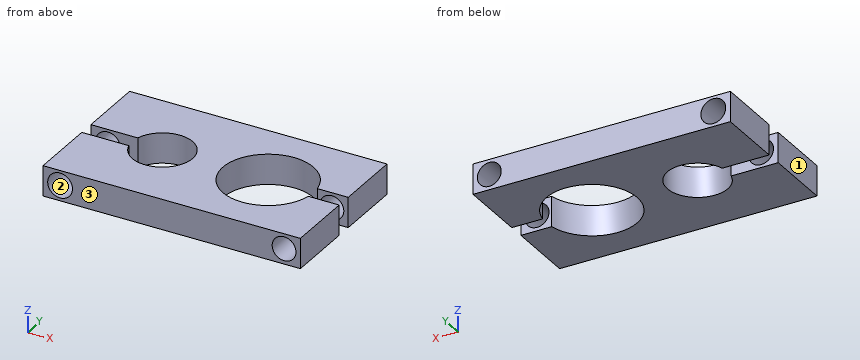
```python
from build123d import *

# Parameters (mm, degrees)
F1_DEPTH = 6.35
F2_R     = 2.607483
F2_R_2   = 2.505418
F3_DEPTH = 34.29


with BuildPart() as f1:
    # F0 (on Top) → F1 (new body)
    with BuildSketch(Plane.XY):
        with BuildLine():
            Line((27.051, 15.875), (-27.051, 15.875))
            Line((-27.051, 15.875), (-27.051, 1.651))
            Line((-27.051, 1.651), (-17.180615, 1.651))
            ThreePointArc((-17.180615, 1.651), (-4.699, 0), (-17.180615, -1.651))
            Line((-17.180615, -1.651), (-27.051, -1.651))
            Line((-27.051, -1.651), (-27.051, -15.875))
            Line((-27.051, -15.875), (27.051, -15.875))
            Line((27.051, -15.875), (27.051, -1.651))
            Line((27.051, -1.651), (20.556822, -1.651))
            ThreePointArc((20.556822, -1.651), (1.651, 0), (20.556822, 1.651))
            Line((20.556822, 1.651), (27.051, 1.651))
            Line((27.051, 1.651), (27.051, 15.875))
        make_face()
    extrude(amount=F1_DEPTH)

    # F2 (on face) → F3 (cut)
    with BuildSketch(Plane.XZ.offset(15.875)):
        with Locations((-23.459613, 3.213262)):
            Circle(F2_R)
        with Locations((23.626484, 3.213262)):
            Circle(F2_R_2)
    extrude(amount=-F3_DEPTH, mode=Mode.SUBTRACT)


solid = f1.part
```
Design review of the part built by this model. Coordinates are the model's own, in mm. Face numbers are marked on the shaded views. Coordinates: 2 decimals unless noted, no trailing zeros. Order: outer loops, then holes, each group sorted by start corner. A loop starts at its lowest first (then second) coordinate and runs counter-clockwise, first axis right, second up. Notation, with made-up numbers: (42, 56.25) -> (70, 56.25) arc R16 ccw to (70, 73.25) -> close; hole circle Ø6 at (44, 85.5). An arc over 180 degrees is marked (long way). One line per item, written item: value. Start each with the question number.
Q1. Take a section at A-A, the plane y = -9. State the section outline as (x, z) points, then the cut area to 3 significant figures.
Q2. Insertion check: pin 1 Ø3 at (x, y) = (-11, -4.5) entering from -Z. The pin has a flat end and moves straight along its axis. Give the tip position at first contact, or say it passes through.
Q3. Mouldability with a two-part tool opening along X and no side actions: class the marked faces 1, 2 and 3 as pulls with the +X half, pulls with the -X half, needs draft (parallel to the pull), parting line crosses it, or undercut.
Q4. Take a section at C-C, the plane z = 4.25. State the section outline as (x, y) points (3 decimals), then the cut area to 3 significant figures.
Q5. Take a section at B-B, the plane x = -19.5. State the section outline as (y, z) points (3 decimals).
Q6. For probe 1 along X at (y, z) = (8.5, 3.5); probe 2 along X at (y, z) = (-11.5, 4.5); probe 3 along X at (y, z) = (-2, 6), list the stretches that pass through material, from the lowest coordinate up.
Q7. Take a section at D-D, the plane y = -4. State the section outline as (x, z) points, then the cut area to 3 significant figures.
Values follow:
1. outline: (-27.05, 0) -> (8.06, 0) -> (8.06, 6.35) -> (-27.05, 6.35) -> close; (14.29, 0) -> (27.05, 0) -> (27.05, 6.35) -> (14.29, 6.35) -> close; hole circle Ø5.21 at (-23.46, 3.21); hole circle Ø5.01 at (23.63, 3.21)
1. area: 263 mm2
2. pin 1: passes through
3. face 1: pulls with the -X half
3. face 2: undercut
3. face 3: needs draft
4. outline: (-27.051, -15.875) -> (-25.852, -15.875) -> (-25.852, -1.651) -> (-27.051, -1.651) -> close; (-27.051, 1.651) -> (-25.852, 1.651) -> (-25.852, 15.875) -> (-27.051, 15.875) -> close; (-21.067, -15.875) -> (21.346, -15.875) -> (21.346, -1.651) -> (20.557, -1.651) arc R9.525 cw (long way) to (20.557, 1.651) -> (21.346, 1.651) -> (21.346, 15.875) -> (-21.067, 15.875) -> (-21.067, 1.651) -> (-17.181, 1.651) arc R6.35 cw (long way) to (-17.181, -1.651) -> (-21.067, -1.651) -> close; (25.907, -15.875) -> (27.051, -15.875) -> (27.051, -1.651) -> (25.907, -1.651) -> close; (25.907, 1.651) -> (27.051, 1.651) -> (27.051, 15.875) -> (25.907, 15.875) -> close
4. area: 987 mm2
5. outline: (-15.875, 0) -> (-1.651, 0) -> (-1.651, 6.35) -> (-15.875, 6.35) -> close; (1.651, 0) -> (15.875, 0) -> (15.875, 6.35) -> (1.651, 6.35) -> close
6. probe 1: x = -27.05 to -26.05, -20.87 to 6.88, 15.47 to 21.14, 26.12 to 27.05
6. probe 2: x = -27.05 to -25.73, -21.19 to 21.48, 25.78 to 27.05
6. probe 3: x = -27.05 to -17.08, -5.02 to 1.86, 20.49 to 27.05
7. outline: (-27.05, 0) -> (-15.98, 0) -> (-15.98, 6.35) -> (-27.05, 6.35) -> close; (-6.12, 0) -> (2.53, 0) -> (2.53, 6.35) -> (-6.12, 6.35) -> close; (19.82, 0) -> (27.05, 0) -> (27.05, 6.35) -> (19.82, 6.35) -> close; hole circle Ø5.21 at (-23.46, 3.21); hole circle Ø5.01 at (23.63, 3.21)
7. area: 130 mm2
